Autodesk Inventor part; units mm, degrees
ref_plane "YZ Plane" through (0, 0, 0) normal (1, 0, 0) x (0, 1, 0)
ref_plane "XZ Plane" through (0, 0, 0) normal (0, 1, 0) x (-1, 0, 0)
ref_plane "XY Plane" through (0, 0, 0) normal (0, 0, 1) x (1, 0, 0)
sketch "Sketch1" plane through (0, 0, 0) normal (0, 0, 1) x (1, 0, 0)
  line L0 (7.6919, 0) -> (-192.3081, 0)
  line L1 (-192.3081, 0) -> (-192.3081, 3)
  line L2 (-192.3081, 3) -> (7.6919, 3)
  line L3 (7.6919, 3) -> (7.6919, 0)
  point P0 (0, 0)
  dimension "d0" = 200
  dimension "d1" = 3
extrude "Extrusion1" add sketch "Sketch1" along normal blind 300
sketch "Sketch2" plane through (-192.3081, 3, 0) normal (0, 1, 0) x (1, 0, 0)
  line L0 (100, -149.5891) -> (200, -149.5891)
  line L1 (200, -149.5891) -> (200, -174.5891)
  line L2 (200, 0) -> (200, -300)
  line L3 (200, -174.5891) -> (100, -174.5891)
  line L4 (200, -149.5891) -> (200, -124.5891)
  line L5 (200, -124.5891) -> (100, -124.5891)
  point P0 (192.3081, 0)
sketch "Sketch3" plane through (-192.3081, 3, 0) normal (0, 1, 0) x (1, 0, 0)
  line L0 (100.0009, -229.5915) -> (100.0009, -174.5915)
  line L1 (100.0089, -124.5986) -> (100.0089, -69.5986)
  line L2 (16.7133, -242.6689) -> (116.7133, -242.6689)
  line L3 (116.7133, -242.6689) -> (116.7133, -281.1334)
  line L4 (116.7133, -281.1334) -> (16.7133, -281.1334)
  line L5 (16.7133, -281.1334) -> (16.7133, -242.6689)
  line L6 (18.3008, -14.1302) -> (116.7133, -14.1302)
  line L7 (116.7133, -14.1302) -> (116.7133, -53.1956)
  line L8 (116.7133, -53.1956) -> (18.3008, -53.1956)
  line L9 (18.3008, -53.1956) -> (18.3008, -14.1302)
  point P0 (192.3081, 0)
extrude "Extrusion2" cut sketch "Sketch3" against normal blind 100
sketch "Sketch4" plane through (-192.3081, 3, 0) normal (0, 1, 0) x (1, 0, 0)
  point P0 (192.3081, 0)
properties part number "base"
Verification items for the finished model (mm, model axes). Round coordinates to 2 decimals unless told otherwise and drop trailing zeros. Order: outer loops, then holes, each group sorted by start corner. A loop starts at its lowest first (then second) coordinate and runs counter-clockwise, first axis right, second up. Notation, with made-up numbers: (86, 16.25) - (137, 16.25) arc R20 cw to (137, 20.25) - close; hole circle Ø7 at (8.5, 61). An arc over 180 degrees is marked (long way). Use CSV: the item, a comma, the result in double quotes. Start each with the question number.
1) Section check A-A, the plane y = 2.35. Record the cut outline in (x, z), plus the area to 3 significant figures.
2) Section check B-B, the plane x = -155.5. Record the cut outline in (y, z).
3) Thickness scan on L1, parallel to Z at x = -147, y = 2.9; L2, parallel to X at y = 0.75, z = 245. Record the ranges inside material, lowest first.
Answers:
1,outline,"(-192.31, 0) - (7.69, 0) - (7.69, 300) - (-192.31, 300) - close; hole (-175.59, 242.67) - (-75.59, 242.67) - (-75.59, 281.13) - (-175.59, 281.13) - close; hole (-174.01, 14.13) - (-75.59, 14.13) - (-75.59, 53.2) - (-174.01, 53.2) - close"
1,area,"52,300 mm²"
2,outline,"(0, 0) - (3, 0) - (3, 14.13) - (0, 14.13) - close; (0, 53.2) - (3, 53.2) - (3, 242.67) - (0, 242.67) - close; (0, 281.13) - (3, 281.13) - (3, 300) - (0, 300) - close"
3,L1,"z = 0 to 14.13, 53.2 to 242.67, 281.13 to 300"
3,L2,"x = -192.31 to -175.59, -75.59 to 7.69"
